from build123d import *

# Parameters (mm, degrees)
SKETCH1_W                      = 84.401025
SKETCH1_H                      = 208.28
BOSS_EXTRUDE1_DEPTH            = 1.905
F_6_CLEARANCE_HOLE1_AT_2_COUNT = 2
F_6_CLEARANCE_HOLE1_AT_2_PITCH = 189.23
F_6_CLEARANCE_HOLE1_AT_3_COUNT = 2
F_6_CLEARANCE_HOLE1_AT_3_PITCH = 201.912164523
F_6_CLEARANCE_HOLE1_AT_4_COUNT = 2
F_6_CLEARANCE_HOLE1_AT_4_PITCH = 70.431025
SKETCH4_W                      = 8.466667
SKETCH4_H                      = 8.466667
BOSS_EXTRUDE2_DEPTH            = 9.525
CUT_EXTRUDE3_DEPTH             = 6.35
CHAMFER1_SIZE                  = 0.635


with BuildPart() as part:
    # Sketch1 → Boss-Extrude1 (new body)
    with BuildSketch(Plane.XY):
        Rectangle(SKETCH1_W, SKETCH1_H)
    extrude(amount=BOSS_EXTRUDE1_DEPTH)

    # Sketch3 → #6 Clearance Hole1 (revolve, cut)
    with BuildSketch(Plane(origin=(-37.7555125, 94.615, 1.905), x_dir=(0, -1, 0), z_dir=(1, 0, 0))):
        Polygon((0, 0), (0, 1.905), (2.15265, 1.905), (2.15265, 1.17475), (3.3274, 0), align=None)
    f_6_clearance_hole1 = revolve(axis=Axis((-37.7555125, 94.615, 8.255), (0, 0, -1)), mode=Mode.SUBTRACT)

    # #6 Clearance Hole1 at 2: #6 Clearance Hole1 ×2
    with Locations(*[(0, -i * F_6_CLEARANCE_HOLE1_AT_2_PITCH, 0) for i in range(1, F_6_CLEARANCE_HOLE1_AT_2_COUNT)]):
        add(f_6_clearance_hole1, mode=Mode.SUBTRACT)

    # #6 Clearance Hole1 at 3: #6 Clearance Hole1 ×2
    with Locations(*[Vector(0.34882011772903904, -0.9371896955619494, 0) * (i * F_6_CLEARANCE_HOLE1_AT_3_PITCH) for i in range(1, F_6_CLEARANCE_HOLE1_AT_3_COUNT)]):
        add(f_6_clearance_hole1, mode=Mode.SUBTRACT)

    # #6 Clearance Hole1 at 4: #6 Clearance Hole1 ×2
    with Locations(*[(i * F_6_CLEARANCE_HOLE1_AT_4_PITCH, 0, 0) for i in range(1, F_6_CLEARANCE_HOLE1_AT_4_COUNT)]):
        add(f_6_clearance_hole1, mode=Mode.SUBTRACT)

    # Sketch4 → Boss-Extrude2 (add)
    with BuildSketch(Plane(origin=(0, 0, 0), x_dir=(-1, 0, 0), z_dir=(0, 0, -1))):
        with Locations((37.967179, -8.0433335)):
            Rectangle(SKETCH4_W, SKETCH4_H)
        with Locations((37.967179, -82.973333082)):
            Rectangle(SKETCH4_W, SKETCH4_H)
    extrude(amount=BOSS_EXTRUDE2_DEPTH)

    # Sketch5 → Cut-Extrude3 (cut)
    with BuildSketch(Plane(origin=(-42.2005125, 0, 0), x_dir=(0, 0, -1), z_dir=(1, 0, 0))):
        Polygon((2.116666667, -82.973333082), (5.291666667, -79.798333082), (8.466666667, -82.973333082), (5.291666667, -86.148333082), align=None)
        Polygon((2.116666667, -8.0433335), (5.291666667, -4.8683335), (8.466666667, -8.0433335), (5.291666667, -11.2183335), align=None)
    extrude(amount=CUT_EXTRUDE3_DEPTH, mode=Mode.SUBTRACT)

    # Chamfer1
    chamfer1_edges = [part.edges().sort_by_distance(p)[0] for p in [
        (-42.2005125, -84.560833082, -3.704166667),
        (-42.2005125, -84.560833082, -6.879166667),
        (-42.2005125, -81.385833082, -6.879166667),
        (-42.2005125, -81.385833082, -3.704166667),
        (-35.8505125, -84.560833082, -3.704166667),
        (-35.8505125, -84.560833082, -6.879166667),
        (-35.8505125, -81.385833082, -6.879166667),
        (-35.8505125, -81.385833082, -3.704166667),
        (-42.2005125, -9.6308335, -3.704166667),
        (-42.2005125, -9.6308335, -6.879166667),
        (-42.2005125, -6.4558335, -6.879166667),
        (-42.2005125, -6.4558335, -3.704166667),
        (-35.8505125, -9.6308335, -3.704166667),
        (-35.8505125, -9.6308335, -6.879166667),
        (-35.8505125, -6.4558335, -6.879166667),
        (-35.8505125, -6.4558335, -3.704166667),
    ]]
    chamfer(chamfer1_edges, length=CHAMFER1_SIZE)


solid = part.part
CAD build for the part. Positions are in the model's coordinates, mm. A direction names the side the tool comes from. Give positions to 0.01 mm unless a question says otherwise; leave off trailing zeros. Loops run counter-clockwise (first coordinate to the right, second up) from the corner with the lowest first, then second, coordinate; pieces in that order, holes last. Notation, with made-up numbers: M -2.5,-36.75 L 28.5,-36.75 A21 cw 28.5,-18.75 Z; hole C 6.25,87 d5. An arc over 180 degrees is marked long. One line per question, with ' | ' between items. Start each with the question number.
1. Two-plate mould, pull along Z, no slides. Class faces 1 (the face through (-41.879, -81.193, -3.454)), 2 (the face through (-38, -83, -9.525)), 3 (the face through (-41.879, -9.824, -7.129)), 4 (the face through (-38, -12.277, -5)): pulls with the +Z half, pulls with the -Z half, needs draft (parallel to the pull), parting line crosses it, or undercut.
2. 3-axis set-ups, long thin cutter, end or side, ignore diameter. For faces 5 (the face through (-38, -87.207, -5)), 6 (the face through (-38, -3.81, -5)), 7 (the face through (-38, -78.74, -5)), 8 (the face through (-41.88, -84.81, -3.51)), 9 (the face through (-33.734, -83, -5)): which of +Z, -Z, +X, -X, +Y, -Y reach the whole face in a straight line?
3. Saw through at A-A on y = 45. Give the cut face in (x, z) (3 decimals).
4. Flat gauge pins, fed straight in: pin 1 (4 mm diameter, centred on x = -38, z = -5, fed in from +Y); pin 2 (4 mm diameter, centred on y = -8, z = -4.5, fed in from +X); pin 3 (2.5 mm diameter, centred on x = -37.76, y = -94.62, fed in from +Z); pin 4 (5.5 mm diameter, centred on x = 32.68, y = -94.61, fed in from -Z). Where does each tip first touch, or does it go through?
5. Saw through at B-B on x = -31. Give the cut face in (y, z) (3 decimals).
6. Probe L1, parallel to Z at x = -28.5, y = 95 (3 decimals). List the from-to ranges inside material, lowest first. Write a range as from..to.
Result sheet:
1) face 1: undercut | face 2: pulls with the -Z half | face 3: undercut | face 4: needs draft
2) face 5: -Z, +X, -X, -Y | face 6: -Z, +X, -X, +Y | face 7: -Z, +X, -X | face 8: -X | face 9: -Z, +X, +Y, -Y
3) outline: M -42.201,0 L 42.201,0 L 42.201,1.905 L -42.201,1.905 Z
4) pin 1: stops at y = -3.81 | pin 2: stops at x = -33.73 | pin 3: passes through | pin 4: stops at z = 0
5) outline: M -104.14,0 L 104.14,0 L 104.14,1.905 L -104.14,1.905 Z
6) L1: z = 0..1.905
